```python
from build123d import *

# Parameters (mm, degrees)
F4_DEPTH = 25
F5_R     = 1.5
F6_DEPTH = 12.5
F8_W     = 10
F8_H     = 3
F9_DEPTH = 2.7


with BuildPart() as f2:
    # F0 (on Right) → F2 (revolve)
    with BuildSketch(Plane.YZ):
        with BuildLine():
            Line((4.6, 10.95), (0, 10.95))
            Line((0, 10.95), (0, 10.2))
            Line((0, 10.2), (7, 10.2))
            Line((7, 10.2), (7, 9.625))
            Line((7, 9.625), (16.7, 9.625))
            Line((16.7, 9.625), (16.7, 0))
            Line((16.7, 0), (29.3, 0))
            Line((29.3, 0), (29.3, 6.1))
            Line((29.3, 6.1), (28.3, 6.1))
            Line((28.3, 6.1), (27.9, 6.6))
            Line((27.9, 6.6), (22.9, 6.6))
            Line((22.9, 6.6), (22.9, 10.95))
            Line((22.9, 10.95), (14.2, 10.95))
            ThreePointArc((14.2, 10.95), (13.7, 10.45), (13.2, 10.95))
            Line((13.2, 10.95), (13.2, 11.15))
            Line((13.2, 11.15), (5.6, 11.15))
            Line((5.6, 11.15), (5.6, 10.95))
            ThreePointArc((5.6, 10.95), (5.1, 10.45), (4.6, 10.95))
        make_face()
    revolve(axis=Axis((0, 2.436379, 0), (0, 1, 0)))

    # F3 (on Front) → F4 (cut)
    with BuildSketch(Plane.XZ):
        Polygon((-0.25, 11.15), (0, 10.95), (0.25, 11.15), (0.25, 11.247457), (-0.25, 11.247457), align=None)
        Polygon((-4.803139, 10.173379), (-4.7635, 10.084348), (-4.453766, 10.003323), (-4.306727, 10.287716), (-4.346367, 10.376747), align=None)
        Polygon((-8.525772, 7.340232), (-8.453347, 7.27502), (-8.137436, 7.32698), (-8.118782, 7.646592), (-8.191207, 7.711804), align=None)
        Polygon((-10.774222, 3.237891), (-10.681534, 3.207775), (-10.414069, 3.383736), (-10.527026, 3.683304), (-10.619713, 3.713419), align=None)
        Polygon((-11.15971, -1.42431), (-11.062787, -1.414123), (-10.890015, -1.144587), (-11.115051, -0.916862), (-11.211974, -0.927049), align=None)
        Polygon((-9.615583, -5.840235), (-9.531183, -5.791506), (-9.482978, -5.475), (-9.781183, -5.358494), (-9.865583, -5.407222), align=None)
        Polygon((-6.408835, -9.24633), (-6.351551, -9.167486), (-6.436249, -8.858736), (-6.75606, -8.873593), (-6.813344, -8.952438), align=None)
        Polygon((-2.093941, -11.053651), (-2.073678, -10.958324), (-2.276633, -10.710716), (-2.562752, -10.854368), (-2.583015, -10.949695), align=None)
        Polygon((2.583015, -10.949695), (2.562752, -10.854368), (2.276633, -10.710716), (2.073678, -10.958324), (2.093941, -11.053651), align=None)
        Polygon((6.813344, -8.952438), (6.75606, -8.873593), (6.436249, -8.858736), (6.351551, -9.167486), (6.408835, -9.24633), align=None)
        Polygon((9.865583, -5.407222), (9.781183, -5.358494), (9.482978, -5.475), (9.531183, -5.791506), (9.615583, -5.840235), align=None)
        Polygon((11.211974, -0.927049), (11.115051, -0.916862), (10.890015, -1.144587), (11.062787, -1.414123), (11.15971, -1.42431), align=None)
        Polygon((10.619713, 3.713419), (10.527026, 3.683304), (10.414069, 3.383736), (10.681534, 3.207775), (10.774222, 3.237891), align=None)
        Polygon((8.191207, 7.711804), (8.118782, 7.646592), (8.137436, 7.32698), (8.453347, 7.27502), (8.525772, 7.340232), align=None)
        Polygon((4.346367, 10.376747), (4.306727, 10.287716), (4.453766, 10.003323), (4.7635, 10.084348), (4.803139, 10.173379), align=None)
    extrude(amount=-F4_DEPTH, mode=Mode.SUBTRACT)

    # F5 (on Right) → F6 (cut, symmetric)
    with BuildSketch(Plane.YZ):
        with Locations((19.7, 8.447273)):
            Circle(F5_R)
    extrude(amount=F6_DEPTH, both=True, mode=Mode.SUBTRACT)

    # F8 (on offset) → F9 (cut)
    with BuildSketch(Plane.XY.offset(11.15)):
        with Locations((6.2, 19.7)):
            Rectangle(F8_W, F8_H)
        with Locations((-6.2, 19.7)):
            Rectangle(F8_W, F8_H)
    extrude(amount=-F9_DEPTH, mode=Mode.SUBTRACT)


solid = f2.part
```
Input: part model. Units: mm. Frame: model coordinates. A direction names the side the tool comes from. Round coordinates to 2 decimals unless told otherwise and drop trailing zeros. Write each loop counter-clockwise with the first axis right and the second up, starting at its lowest first coordinate (ties: lowest second). Pieces come first, ordered by that corner, then holes. Notation, with made-up numbers: M 26,-27.75 L 40,-27.75 A27 cw 40,-5.75 Z; hole C 88.5,80.25 d11. An arc over 180 degrees is marked long. Write each question's results on one line, items separated by ' | '.
Q1. Section query A-A (y = 19.7). Return loops of the section in (x, z).
Results:
outline: M -8.46,6.95 A10.95 ccw long 8.46,6.95 Z; M -1.2,9.95 L 1.2,9.95 L 1.2,10.88 A10.95 ccw -1.2,10.88 Z
Q2. Section query C-C (y = 2.5). Return loops of the section in (x, z), and give its area (3 significant figures).
Results:
outline: C 0,0 d21.9; hole C 0,0 d20.4 | area: 49.8 mm^2
Q3. Draft query along Y for faces 4 (the face through (11.086, 9.347, 1.195)), 5 (the face through (-3, 18.2, 9)), 6 (the face through (-8, 7, -6)), 7 (the face through (3, 18.2, 9)). Return one class per face: released by +Y, released by -Y, zero draft, split by the parting line, or undercut.
Results:
face 4: zero draft | face 5: undercut | face 6: released by -Y | face 7: undercut
Q4. Access query for faces 1 (the face through (4.461, 25.365, -4.864)), 2 (the face through (1.2, 19.7, 10.2)), 3 (the face through (-6.66, 2.27, -8.69)). Directions: +Z, -Z, +X, -X, +Y, -Y. A direction counts if a zero-diameter tool reaches every point of the face in a straight line with its end or side. Return the directions, or none.
Results:
face 1: +Y | face 2: +Z, +X | face 3: -Y
Q5. Line query: line 1 along X through (y, z) = (9.5, 0) (3 decimals); line 2 along X through (y, z) = (5.75, 0); line 3 along Y through (x, z) = (-3.75, 8.75). Output: solid intervals per line, ascending.
Results:
line 1: x = -11.15 to -9.625, 9.625 to 11.15 | line 2: x = -11.15 to -10.2, 10.2 to 11.15 | line 3: y = 16.7 to 18.2, 21.2 to 22.9
Q6. Pin query (flat end, axial travel): P1, Ø2, axis at x = -8.5, z = -3.5, coming from the +Y side; P2, Ø8, axis at x = -3, z = 8, coming from the -Y side; P3, Ø1.5, axis at x = -2, z = 7, coming from the -Y side; P4, Ø4, axis at x = -8.5, y = 14, coming from the +Z side. Return the tip coordinate at first contact, or that it passes through.
Results:
P1: stops at y = 22.9 | P2: stops at y = 0 | P3: stops at y = 16.7 | P4: stops at z = 8.94
